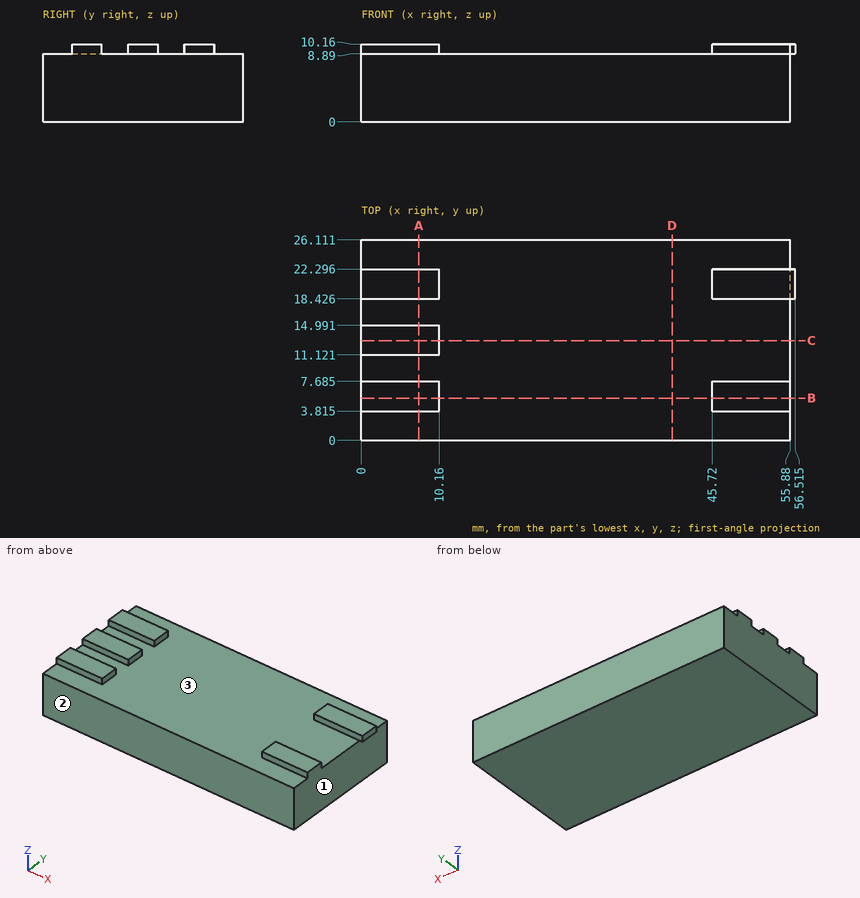
Design review of the part shown in the three views and the two pictorial views. Dimensions are in mm from the part's minimum x, y and z. Coordinates: 2 decimals unless noted, no trailing zeros. Loops run counter-clockwise (first coordinate to the right, second up) from the corner with the lowest first, then second, coordinate; pieces in that order, holes last. Notation, with made-up numbers: M -39.5,-0.5 L -18.5,-0.5 A24 ccw -18.5,24.5 Z; hole C 42,27.5 d6. An arc over 180 degrees is marked long. Put each result on its own line as item: value. Start each with the question number.
Q1. Add section D-D (x = 40.5). Write out the cut boundary in (y, z), and give its area (3 significant figures).
Q2. Add section A-A (x = 7.5). Write out the cut boundary in (y, z) (1 decimal), and give its area (3 significant figures).
Q3. Add section C-C (y = 13). Write out the cut boundary in (x, z), and give its area (3 significant figures).
Q4. Add section B-B (y = 5.5). Write out the cut boundary in (x, z).
Q5. The part is to be moulded in two halves that separate along X. For the marked faces 1, 2 and 3, say which applies: +X half, -X half, draft (parallel to the pull), parting line (faces both ways), or undercut.
Q6. Wall thickness on line 1 (X direction, y = 19.75, z = 9.25) (1 decimal); line 2 (Y direction, x = 47.5, z = 9) (1 decimal); line 3 (Z direction, x = 43, y = 23.75): over which ranges is each line inside the solid? List them lowest first.
Q7. Clearance check with flat-ended pins moving along their axes: pin 1 (1 mm diameter, centred on x = 4, z = 9.5, fed in from +Y); pin 2 (1 mm diameter, centred on x = 7.5, z = 9.5, fed in from -Y) (1 decimal); pin 3 (1 mm diameter, centred on y = 6, z = 9.5, fed in from +X). State where each tip first meets the part, or that it passes through.
Answers:
1. outline: M 0,0 L 26.11,0 L 26.11,8.89 L 0,8.89 Z
1. area: 232 mm^2
2. outline: M 0,0 L 26.1,0 L 26.1,8.9 L 22.3,8.9 L 22.3,10.2 L 18.4,10.2 L 18.4,8.9 L 15,8.9 L 15,10.2 L 11.1,10.2 L 11.1,8.9 L 7.7,8.9 L 7.7,10.2 L 3.8,10.2 L 3.8,8.9 L 0,8.9 Z
2. area: 247 mm^2
3. outline: M 0,0 L 55.88,0 L 55.88,8.89 L 10.16,8.89 L 10.16,10.16 L 0,10.16 Z
3. area: 510 mm^2
4. outline: M 0,0 L 55.88,0 L 55.88,10.16 L 45.72,10.16 L 45.72,8.89 L 10.16,8.89 L 10.16,10.16 L 0,10.16 Z
5. face 1: +X half
5. face 2: draft
5. face 3: undercut
6. line 1: x = 0 to 10.2, 45.7 to 56.5
6. line 2: y = 3.8 to 7.7, 18.4 to 22.3
6. line 3: z = 0 to 8.89
7. pin 1: stops at y = 22.3
7. pin 2: stops at y = 3.8
7. pin 3: stops at x = 55.88
